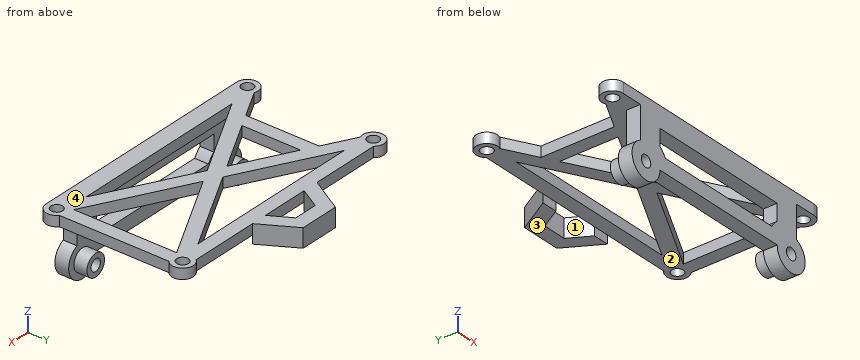
```python
from build123d import *

# Parameters (mm, degrees)
SKETCH1_R           = 1.7
BOSS_EXTRUDE1_DEPTH = 3
SKETCH2_R           = 1.7
BOSS_EXTRUDE2_DEPTH = 4
BOSS_EXTRUDE3_START = -4
SKETCH2_3_R         = 3.15
SKETCH2_3_R_2       = 1.7
BOSS_EXTRUDE3_DEPTH = 3.8
BOSS_EXTRUDE4_DEPTH = 2.4


with BuildPart() as part:
    # Sketch1 → Boss-Extrude1 (new body)
    with BuildSketch(Plane.XY):
        with BuildLine():
            Line((-33.013012558, 15.364996561), (-24.16, 10.636565235))
            Line((-24.16, 10.636565235), (-24.16, -10.636565235))
            Line((-24.16, -10.636565235), (-33.013012558, -15.364996561))
            ThreePointArc((-33.013012558, -15.364996561), (-37.204504119, -17.661052511), (-34.16, -21.345))
            Line((-34.16, -21.345), (34.16, -21.345))
            ThreePointArc((34.16, -21.345), (37.071398801, -19.30978027), (36.16, -15.876456144))
            Line((36.16, -15.876456144), (36.16, 15.876456144))
            ThreePointArc((36.16, 15.876456144), (36.352031022, 20.437031022), (31.791456144, 20.245))
            Line((31.791456144, 20.245), (11.547005384, 20.245))
            Line((11.547005384, 20.245), (5.773502692, 30.245))
            Line((5.773502692, 30.245), (-5.773502692, 30.245))
            Line((-5.773502692, 30.245), (-11.547005384, 20.245))
            Line((-11.547005384, 20.245), (-31.791456144, 20.245))
            ThreePointArc((-31.791456144, 20.245), (-37.167216066, 18.9977626), (-33.013012558, 15.364996561))
        make_face()
        Polygon((32.16, -14.909398958), (4.24522508, 0), (32.16, 14.909398958), align=None, mode=Mode.SUBTRACT)
        Polygon((6.92820323, 20.245), (-6.92820323, 20.245), (-3.464101615, 26.245), (3.464101615, 26.245), align=None, mode=Mode.SUBTRACT)
        Polygon((-4.24522508, 0), (-20.16, -8.500148373), (-20.16, 8.500148373), align=None, mode=Mode.SUBTRACT)
        Polygon((26.170187362, -16.245), (-26.170187362, -16.245), (0, -2.267392611), align=None, mode=Mode.SUBTRACT)
        Polygon((0, 2.267392611), (-26.170187362, 16.245), (26.170187362, 16.245), align=None, mode=Mode.SUBTRACT)
        with Locations((-34.16, 18.245)):
            Circle(SKETCH1_R, mode=Mode.SUBTRACT)
        with Locations((-34.16, -18.245)):
            Circle(SKETCH1_R, mode=Mode.SUBTRACT)
        with Locations((34.16, -18.245)):
            Circle(SKETCH1_R, mode=Mode.SUBTRACT)
        with Locations((34.16, 18.245)):
            Circle(SKETCH1_R, mode=Mode.SUBTRACT)
    extrude(amount=-BOSS_EXTRUDE1_DEPTH)

    # Sketch2 → Boss-Extrude2 (add)
    with BuildSketch(Plane.XZ.offset(21.345)):
        with BuildLine():
            Line((-28, -3), (-28, -12.417424305))
            ThreePointArc((-28, -12.417424305), (-28.738612788, -21.183300133), (-21, -17))
            Line((-21, -17), (21, -17))
            ThreePointArc((21, -17), (28.738612788, -21.183300133), (28, -12.417424305))
            Line((28, -12.417424305), (28, -3))
            Line((28, -3), (-28, -3))
        make_face()
        with BuildLine():
            Line((19.07179677, -13), (-19.07179677, -13))
            ThreePointArc((-19.07179677, -13), (-19.931185282, -11.787564109), (-21, -10.755002002))
            Line((-21, -10.755002002), (-21, -6))
            Line((-21, -6), (21, -6))
            Line((21, -6), (21, -10.755002002))
            ThreePointArc((21, -10.755002002), (19.931185282, -11.787564109), (19.07179677, -13))
        make_face(mode=Mode.SUBTRACT)
        with Locations((-26, -17)):
            Circle(SKETCH2_R, mode=Mode.SUBTRACT)
        with Locations((26, -17)):
            Circle(SKETCH2_R, mode=Mode.SUBTRACT)
    extrude(amount=-BOSS_EXTRUDE2_DEPTH)

    # Sketch2<3> → Boss-Extrude3 (add)
    with BuildSketch(Plane.XZ.offset(21.345).offset(BOSS_EXTRUDE3_START)):
        with Locations((-26, -17)):
            Circle(SKETCH2_3_R)
        with Locations((-26, -17)):
            Circle(SKETCH2_3_R_2, mode=Mode.SUBTRACT)
        with Locations((26, -17)):
            Circle(SKETCH2_3_R)
        with Locations((26, -17)):
            Circle(SKETCH2_3_R_2, mode=Mode.SUBTRACT)
    extrude(amount=-BOSS_EXTRUDE3_DEPTH)

    # Sketch3 → Boss-Extrude4 (add)
    with BuildSketch(Plane(origin=(0, 0, -3), x_dir=(-1, 0, 0), z_dir=(0, 0, -1))):
        Polygon((-3.464101615, 26.245), (3.464101615, 26.245), (6.92820323, 20.245), (11.547005384, 20.245), (5.773502692, 30.245), (-5.773502692, 30.245), (-11.547005384, 20.245), (-6.92820323, 20.245), align=None)
    extrude(amount=BOSS_EXTRUDE4_DEPTH)


solid = part.part
```
For this review, take the finished solid that the model builds, in its own axes (mm). Face numbers are marked on the shaded views. A direction names the side the tool comes from. Round coordinates to 2 decimals unless told otherwise and drop trailing zeros. Loops run counter-clockwise (first coordinate to the right, second up) from the corner with the lowest first, then second, coordinate; pieces in that order, holes last.
Q1. Machinability: for the marked faces 3 and 4, which of the approach directions +Z, -Z, +X, -X, +Y, -Y give a long, thin tool a straight path to every point of the face, cutting with its end or side? Answer none if there is none.
Result sheet:
face 3: -Z, +X, -X, +Y
face 4: +Z, +X, -X, +Y, -Y
Q2. Add section B-B on y = -6.5. Write out the cut boundary in (x, z).
Result sheet:
outline: (-24.16, -3) - (-20.16, -3) - (-20.16, 0) - (-24.16, 0) - close; (-16.42, -3) - (-7.92, -3) - (-7.92, 0) - (-16.42, 0) - close; (7.92, -3) - (16.42, -3) - (16.42, 0) - (7.92, 0) - close; (32.16, -3) - (36.16, -3) - (36.16, 0) - (32.16, 0) - close
Q3. Insertion check: pin 1 Ø0.9 at (y, z) = (6, -1.5) entering from -X; pin 2 Ø11 at (x, y) = (4.5, 27) entering from -Z; pin 3 Ø2 at (y, z) = (-20.5, -6.5) entering from +X; pin 4 Ø10 at (y, z) = (8, -8.5) entering from -X. Each pin has a flat end and moves straight along its axis. Give the tip position at first contact, or say it passes through.
Result sheet:
pin 1: stops at x = -24.16
pin 2: stops at z = -5.4
pin 3: stops at x = 28
pin 4: passes through
Q4. Add section D-D on z = -4.25. Write out the cut boundary in (x, y) (1 decimal), plus the area to 3 significant figures.
Result sheet:
outline: (-28, -21.3) - (28, -21.3) - (28, -17.3) - (-28, -17.3) - close; (-11.5, 20.2) - (-6.9, 20.2) - (-3.5, 26.2) - (3.5, 26.2) - (6.9, 20.2) - (11.5, 20.2) - (5.8, 30.2) - (-5.8, 30.2) - close
area: 335 mm2
Q5. Add section A-A on z = -7.75. Write out the cut boundary in (x, y) (3 decimals), plus the area to 3 significant figures.
Result sheet:
outline: (-28, -21.345) - (-21, -21.345) - (-21, -17.345) - (-28, -17.345) - close; (21, -21.345) - (28, -21.345) - (28, -17.345) - (21, -17.345) - close
area: 56.0 mm2
Q6. Add section C-C on x = -17. Write out the cut boundary in (y, z) (3 decimals), plus the area to 3 significant figures.
Result sheet:
outline: (-21.345, -17) - (-17.345, -17) - (-17.345, -13) - (-21.345, -13) - close; (-21.345, -6) - (-17.345, -6) - (-17.345, -3) - (-16.245, -3) - (-16.245, 0) - (-21.345, 0) - close; (-11.347, -3) - (-6.812, -3) - (-6.812, 0) - (-11.347, 0) - close; (6.812, -3) - (11.347, -3) - (11.347, 0) - (6.812, 0) - close; (16.245, -3) - (20.245, -3) - (20.245, 0) - (16.245, 0) - close
area: 82.5 mm2
Q7. To check wall thickness, follow line 1 along Y through (x, z) = (34.16, -0.6) (3 decimals); line 2 along Y through (x, z) = (-34.16, -0.65) (3 decimals); line 3 along X through (y, z) = (20.5, -1.75). State the ranges of each line that lie inside material, in increasing order.
Result sheet:
line 1: y = -21.345 to -19.945, -16.545 to 16.545, 19.945 to 21.345
line 2: y = -21.345 to -19.945, -16.545 to -15.145, 15.145 to 16.545, 19.945 to 21.345
line 3: x = -36.29 to -32.03, -11.4 to -6.78, 6.78 to 11.4, 32.03 to 36.29
Q8. Mouldability with a two-part tool opening along X and no side actions: class the marked faces 1 and 2 as +X half, -X half, draft (parallel to the pull), parting line (faces both ways), or undercut.
Result sheet:
face 1: undercut
face 2: draft
